Model file for the job. Use its own axes, mm. Round coordinates to 2 decimals unless told otherwise and drop trailing zeros. Answer as a JSON object with one key per item and string values. Group by question number.
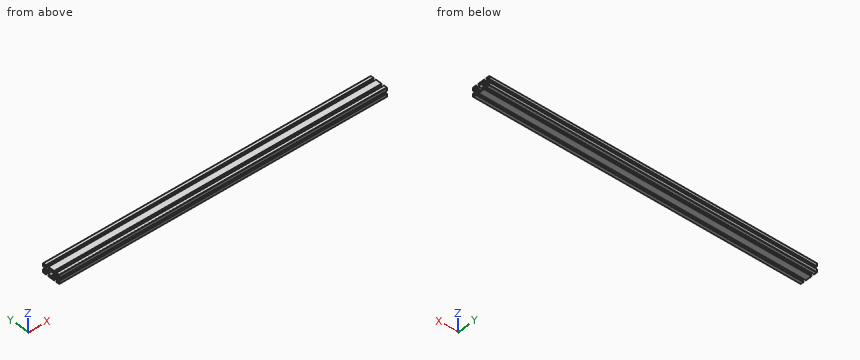
from build123d import *

# Parameters (mm, degrees)
SKETCH1_R           = 2.1
BOSS_EXTRUDE1_DEPTH = 714


with BuildPart() as part:
    # Sketch1 → Boss-Extrude1 (new body)
    with BuildSketch(Plane(origin=(0, 0, 0), x_dir=(0, 0, -1), z_dir=(1, 0, 0))):
        with BuildLine():
            Line((-10, -13), (-10, -19))
            ThreePointArc((-10, -19), (-9.707106781, -19.707106781), (-9, -20))
            Line((-9, -20), (-3, -20))
            Line((-3, -20), (-3, -18))
            Line((-3, -18), (-6, -18))
            Line((-6, -18), (-6, -17.060660172))
            Line((-6, -17.060660172), (-2.939339828, -14))
            Line((-2.939339828, -14), (2.939339828, -14))
            Line((2.939339828, -14), (6, -17.060660172))
            Line((6, -17.060660172), (6, -18))
            Line((6, -18), (3, -18))
            Line((3, -18), (3, -20))
            Line((3, -20), (9, -20))
            ThreePointArc((9, -20), (9.707106781, -19.707106781), (10, -19))
            Line((10, -19), (10, -13))
            Line((10, -13), (8, -13))
            Line((8, -13), (8, -16))
            Line((8, -16), (7.060660172, -16))
            Line((7.060660172, -16), (4, -12.939339828))
            Line((4, -12.939339828), (4, -7.060660172))
            Line((4, -7.060660172), (7.060660172, -4))
            Line((7.060660172, -4), (8, -4))
            Line((8, -4), (8, -7))
            Line((8, -7), (10, -7))
            Line((10, -7), (10, 7))
            Line((10, 7), (8, 7))
            Line((8, 7), (8, 4))
            Line((8, 4), (7.060660172, 4))
            Line((7.060660172, 4), (4, 7.060660172))
            Line((4, 7.060660172), (4, 12.939339828))
            Line((4, 12.939339828), (7.060660172, 16))
            Line((7.060660172, 16), (8, 16))
            Line((8, 16), (8, 13))
            Line((8, 13), (10, 13))
            Line((10, 13), (10, 19))
            ThreePointArc((10, 19), (9.707106781, 19.707106781), (9, 20))
            Line((9, 20), (3, 20))
            Line((3, 20), (3, 18))
            Line((3, 18), (6, 18))
            Line((6, 18), (6, 17.060660172))
            Line((6, 17.060660172), (2.939339828, 14))
            Line((2.939339828, 14), (-2.939339828, 14))
            Line((-2.939339828, 14), (-6, 17.060660172))
            Line((-6, 17.060660172), (-6, 18))
            Line((-6, 18), (-3, 18))
            Line((-3, 18), (-3, 20))
            Line((-3, 20), (-9, 20))
            ThreePointArc((-9, 20), (-9.707106781, 19.707106781), (-10, 19))
            Line((-10, 19), (-10, 13))
            Line((-10, 13), (-8, 13))
            Line((-8, 13), (-8, 16))
            Line((-8, 16), (-7.060660172, 16))
            Line((-7.060660172, 16), (-4, 12.939339828))
            Line((-4, 12.939339828), (-4, 7.060660172))
            Line((-4, 7.060660172), (-7.060660172, 4))
            Line((-7.060660172, 4), (-8, 4))
            Line((-8, 4), (-8, 7))
            Line((-8, 7), (-10, 7))
            Line((-10, 7), (-10, -7))
            Line((-10, -7), (-8, -7))
            Line((-8, -7), (-8, -4))
            Line((-8, -4), (-7.060660172, -4))
            Line((-7.060660172, -4), (-4, -7.060660172))
            Line((-4, -7.060660172), (-4, -12.939339828))
            Line((-4, -12.939339828), (-7.060660172, -16))
            Line((-7.060660172, -16), (-8, -16))
            Line((-8, -16), (-8, -13))
            Line((-8, -13), (-10, -13))
        make_face()
        with Locations((0, 10)):
            Circle(SKETCH1_R, mode=Mode.SUBTRACT)
        with Locations((0, -10)):
            Circle(SKETCH1_R, mode=Mode.SUBTRACT)
        with BuildLine():
            Line((-8, 1.7), (-8, -1.7))
            ThreePointArc((-8, -1.7), (-7.912132034, -1.912132034), (-7.7, -2))
            Line((-7.7, -2), (-7.063603897, -2))
            ThreePointArc((-7.063603897, -2), (-6.948798867, -2.02283614), (-6.851471863, -2.087867966))
            Line((-6.851471863, -2.087867966), (-2.939339828, -6))
            Line((-2.939339828, -6), (2.939339828, -6))
            Line((2.939339828, -6), (6.851471863, -2.087867966))
            ThreePointArc((6.851471863, -2.087867966), (6.948798867, -2.02283614), (7.063603897, -2))
            Line((7.063603897, -2), (7.7, -2))
            ThreePointArc((7.7, -2), (7.912132034, -1.912132034), (8, -1.7))
            Line((8, -1.7), (8, 1.7))
            ThreePointArc((8, 1.7), (7.912132034, 1.912132034), (7.7, 2))
            Line((7.7, 2), (7.063603897, 2))
            ThreePointArc((7.063603897, 2), (6.948798867, 2.02283614), (6.851471863, 2.087867966))
            Line((6.851471863, 2.087867966), (2.939339828, 6))
            Line((2.939339828, 6), (-2.939339828, 6))
            Line((-2.939339828, 6), (-6.851471863, 2.087867966))
            ThreePointArc((-6.851471863, 2.087867966), (-6.948798867, 2.02283614), (-7.063603897, 2))
            Line((-7.063603897, 2), (-7.7, 2))
            ThreePointArc((-7.7, 2), (-7.912132034, 1.912132034), (-8, 1.7))
        make_face(mode=Mode.SUBTRACT)
    extrude(amount=BOSS_EXTRUDE1_DEPTH)


solid = part.part
(1) Slice it at A-A (x = 78). Count the separate pieces of the cut face and the enclosed holes in it, then the cut area to 3 significant figures.
(2) Drill centre lines: line 1 (Y direction, x = 669, z = -7.75); line 2 (Y direction, x = 210, z = 0); line 3 (Z direction, x = 403, y = 1). Where is each one in solid material? Low to high. Write a range as from..to.
(3) Flat gauge pin, fed straight in: pin 1 (3 mm diameter, centred on x = 476, z = 1, fed in from -Y). Where does the tip first touch, or does it go through?
Answer:
{
 "1": {"separate pieces": "1", "enclosed holes": "3", "area": "325 mm²"},
 "2": {"line 1": "-20..-16, -4..-2, 2..4, 16..20", "line 2": "-14..-12.1, -7.9..-6, 6..7.9, 12.1..14", "line 3": "-10..-8, 8..10"},
 "3": {"pin 1": "y = -14"}
}
